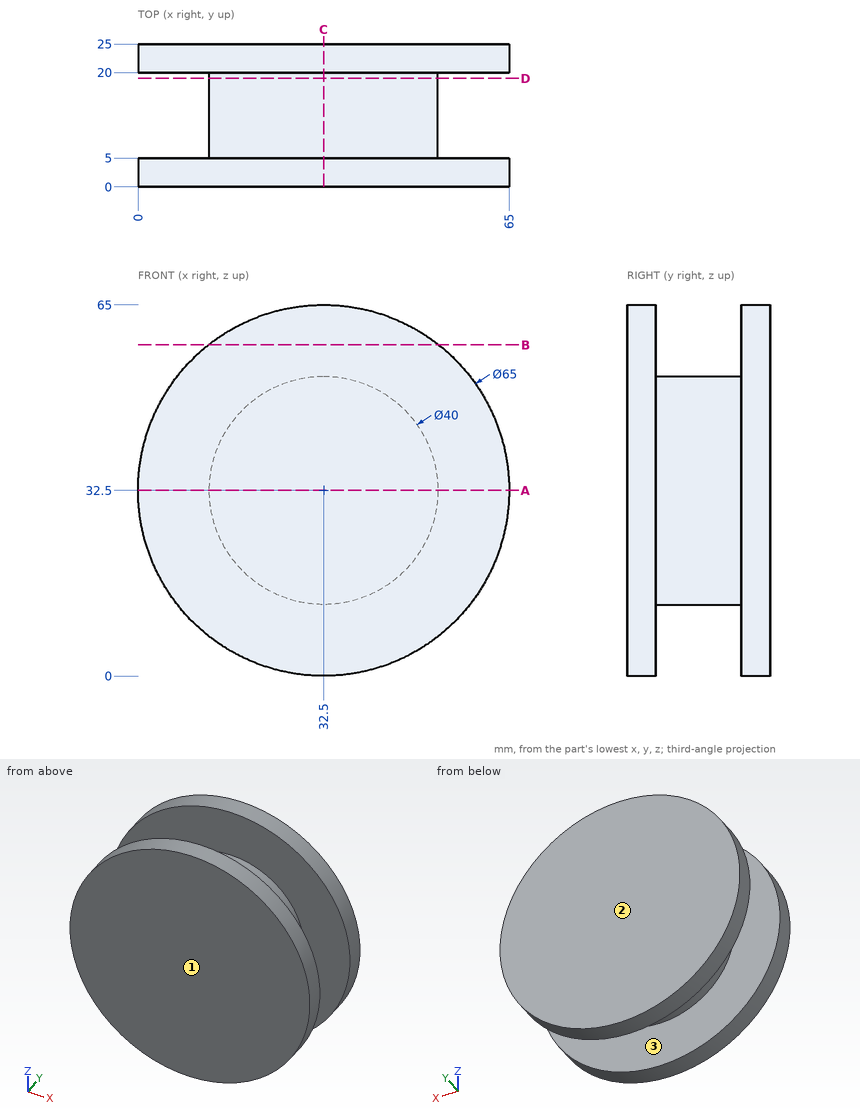
Answer from the drawing. Dimensions are ordinates in mm from the lowest x, y and z of the part. Give positions to 0.01 mm unless a question says otherwise; leave off trailing zeros. Write each loop counter-clockwise with the first axis right and the second up, starting at its lowest first coordinate (ties: lowest second). Pieces come first, ordered by that corner, then holes.
1) Section B-B (z = 58) is taken. Write down the section's boundary in (x, y), and give its area (3 significant figures).
2) For a pull along Y with two mould halves and no side action, classify the marked faces 1, 2 and 3 as pulls with the +Y half, pulls with the -Y half, needs draft (parallel to the pull), parting line crosses it, or undercut.
3) Section D-D (y = 19) is taken. Write down the section's boundary in (x, z), and give its area (3 significant figures).
4) Given P1, Ø12, axis at x = 17, z = 58, coming from the -Y side; P2, Ø2, axis at y = 4.5, z = 28, coming from the -X side; P3, Ø8, axis at y = 5, z = 36.5, coming from the -X side; P4, Ø3, axis at x = 19, y = 16.5, coming from the +Z side, each flat-ended and moving along its own axis, determine where each tip first touches the part or whether it passes through.
5) Section A-A (z = 32.5) is taken. Write down the section's boundary in (x, y), and give its area (3 significant figures).
6) Find the intervals of material crossed by L1, parallel to Y at x = 50.5, z = 21; L2, parallel to Z at x = 33, y = 20.25; L3, parallel to X at y = 22, z = 7, in increasing order.
7) Section C-C (x = 32.5) is taken. Write down the section's boundary in (y, z), and give its area (3 significant figures).
Response:
1. outline: (12.35, 0) - (52.65, 0) - (52.65, 5) - (12.35, 5) - close; (12.35, 20) - (52.65, 20) - (52.65, 25) - (12.35, 25) - close
1. area: 403 mm2
2. face 1: pulls with the -Y half
2. face 2: pulls with the +Y half
2. face 3: undercut
3. outline: circle Ø40 at (32.5, 32.5)
3. area: 1,260 mm2
4. P1: stops at y = 0
4. P2: stops at x = 0.19
4. P3: stops at x = 0
4. P4: stops at z = 48.5
5. outline: (0, 0) - (65, 0) - (65, 5) - (52.5, 5) - (52.5, 20) - (65, 20) - (65, 25) - (0, 25) - (0, 20) - (12.5, 20) - (12.5, 5) - (0, 5) - close
5. area: 1,250 mm2
6. L1: y = 0 to 5, 20 to 25
6. L2: z = 0 to 65
6. L3: x = 12.35 to 52.65
7. outline: (0, 0) - (5, 0) - (5, 12.5) - (20, 12.5) - (20, 0) - (25, 0) - (25, 65) - (20, 65) - (20, 52.5) - (5, 52.5) - (5, 65) - (0, 65) - close
7. area: 1,250 mm2
